Can you work these out from the model? Positions are in its coordinate system, mm. Face numbers are marked on the shaded views. Round coordinates to 2 decimals unless told otherwise and drop trailing zeros. Order: outer loops, then holes, each group sorted by start corner. A loop starts at its lowest first (then second) coordinate and runs counter-clockwise, first axis right, second up. Notation, with made-up numbers: M 62,-15 L 104,-15 A12 ccw 104,-2 Z; hole C 22,1 d10. An arc over 180 degrees is marked long. One line per question, with ' | ' between items.
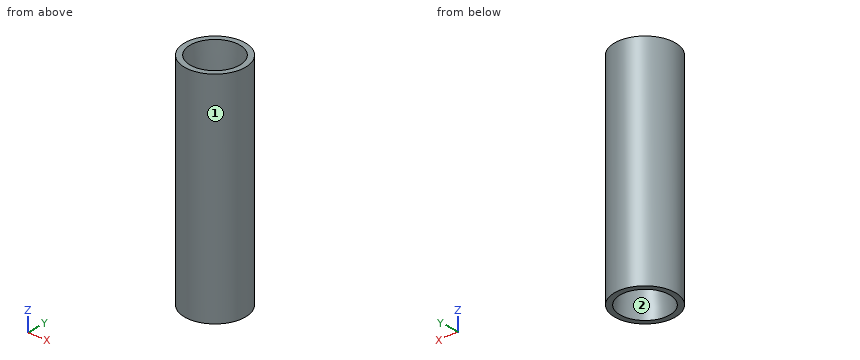
```python
from build123d import *

# Parameters (mm, degrees)
SKETCH1_R           = 2.775
BOSS_EXTRUDE1_DEPTH = 20
SKETCH2_R           = 2.27
CUT_EXTRUDE1_DEPTH  = 5.68
CUT_EXTRUDE1_TAPER  = 3.074
SKETCH7_R           = 1
CUT_EXTRUDE2_DEPTH  = 21
SKETCH9_R           = 2.27
CUT_EXTRUDE3_DEPTH  = 5.68
CUT_EXTRUDE3_TAPER  = 3.074


with BuildPart() as part:
    # Sketch1 → Boss-Extrude1 (new body)
    with BuildSketch(Plane.XY):
        Circle(SKETCH1_R)
    extrude(amount=BOSS_EXTRUDE1_DEPTH)

    # Sketch2 → Cut-Extrude1 (cut)
    with BuildSketch(Plane.XY):
        Circle(SKETCH2_R)
    extrude(amount=CUT_EXTRUDE1_DEPTH, taper=CUT_EXTRUDE1_TAPER, mode=Mode.SUBTRACT)

    # Sketch7 → Cut-Extrude2 (cut, through all)
    with BuildSketch(Plane.XY):
        Circle(SKETCH7_R)
    extrude(amount=CUT_EXTRUDE2_DEPTH, mode=Mode.SUBTRACT)

    # Sketch9 → Cut-Extrude3 (cut)
    with BuildSketch(Plane.XY.offset(20)):
        Circle(SKETCH9_R)
    extrude(amount=-CUT_EXTRUDE3_DEPTH, taper=CUT_EXTRUDE3_TAPER, mode=Mode.SUBTRACT)


solid = part.part
```
(1) If we section it at A-A on x = 0: Please give me the cut outline in (y, z) (3 decimals).
Final values:
outline: M -2.775,0 L -2.27,0 L -1.965,5.68 L -1,5.68 L -1,14.32 L -1.965,14.32 L -2.27,20 L -2.775,20 Z; M 1,5.68 L 1.965,5.68 L 2.27,0 L 2.775,0 L 2.775,20 L 2.27,20 L 1.965,14.32 L 1,14.32 Z
(2) If we section it at C-C on y = 2.45: Please give me the cut outline in (x, z).
Final values:
outline: M -1.3,0 L 1.3,0 L 1.3,20 L -1.3,20 Z
(3) Thinking about a two-plate mould opening in Y: for the marked faces 1 and 2, which applies, released by +Y, released by -Y, zero draft, split by the parting line, or undercut?
Final values:
face 1: split by the parting line | face 2: undercut
(4) Please list where these lines run through material, in increasing order: probe 1 along Y at (x, z) = (0, 11.75) (3 decimals); probe 2 along Y at (x, z) = (-0.1, 15.5); probe 3 along Z at (x, y) = (1.2, 1.35). Write a range as [from, to].
Final values:
probe 1: [-2.775, -1], [1, 2.775] | probe 2: [-2.77, -2.03], [2.03, 2.77] | probe 3: [5.68, 14.32]
(5) Will these pins go through, and if not, where does the flat tip stop? pin 1 Ø2.5 at (x, y) = (0, 0) entering from -Z; pin 2 Ø2 at (x, y) = (0, -0.5) entering from +Z; pin 3 Ø1.5 at (x, y) = (0, 0) entering from +Z.
Final values:
pin 1: z = 5.68 | pin 2: z = 14.32 | pin 3: through
(6) If we section it at D-D on z = 16.75: Please give me the cut outline in (x, y) (3 decimals).
Final values:
outline: C 0,0 d5.55; hole C 0,0 d4.191
(7) If we section it at B-B on z = 8.5: Please give me the cut outline in (x, y) (3 decimals).
Final values:
outline: C 0,0 d5.55; hole C 0,0 d2
